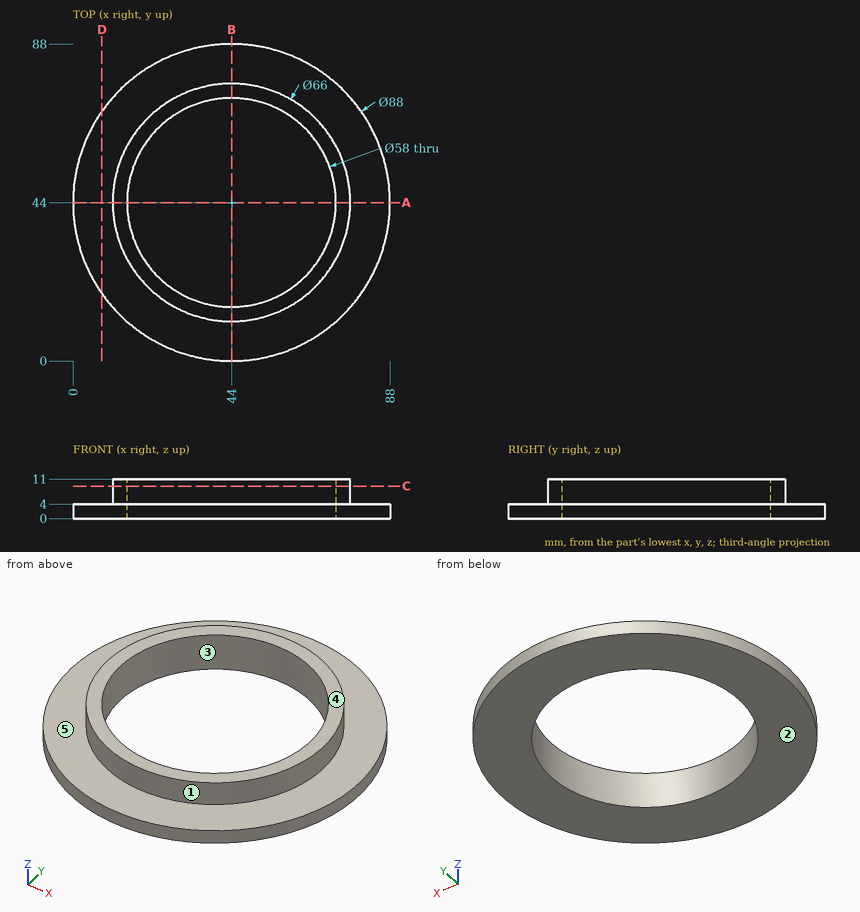
For this review, use the dimensioned drawing (mm, ordinates from the lowest corner) and the shaded views. A direction names the side the tool comes from. Coordinates: 2 decimals unless noted, no trailing zeros. Loops run counter-clockwise (first coordinate to the right, second up) from the corner with the lowest first, then second, coordinate; pieces in that order, holes last.
1. Add section D-D, the plane x = 8. Give the boundary of the cut face in (y, z), then the cut area to 3 significant figures.
2. Insertion check: P1, Ø4, axis at x = 72.5, y = 16, coming from the +Z side; P2, Ø1.5, axis at x = 16, y = 66.5, coming from the -Z side; P3, Ø4, axis at y = 23, z = 1.5, coming from the -X side; P4, Ø6, axis at y = 60.5, z = 7.5, coming from the -X side. Each pin has a flat end and moves straight along its axis. Give the tip position at first contact, or say it passes through.
3. Add section C-C, the plane z = 9. Give the boundary of the cut face in (x, y), then the cut area to 3 significant figures.
4. Mouldability with a two-part tool opening along X and no side actions: class the marked faces 1, 2 and 3 as +X half, -X half, draft (parallel to the pull), parting line (faces both ways), or undercut.
5. Add section A-A, the plane y = 44. Give the boundary of the cut face in (x, z), then the cut area to 3 significant figures.
6. For line 1 (Z direction, x = 7.5, y = 59.5); line 2 (Y direction, x = 32, z = 2.5); line 3 (Y direction, x = 44, z = 2), list the stretches that pass through material, from the lowest coordinate up.
7. For the marked faces 4 and 5, list the 3-axis set-ups (+Z, -Z, +X, -X, +Y, -Y) from which the entire face can be reached by the end or side of a thin tool; tool diameter is ignored.
Result:
1. outline: (18.7, 0) - (69.3, 0) - (69.3, 4) - (18.7, 4) - close
1. area: 202 mm2
2. P1: stops at z = 4
2. P2: stops at z = 0
2. P3: stops at x = 4.31
2. P4: stops at x = 13.89
3. outline: circle Ø66 at (44, 44); hole circle Ø58 at (44, 44)
3. area: 779 mm2
4. face 1: parting line
4. face 2: draft
4. face 3: undercut
5. outline: (0, 0) - (15, 0) - (15, 11) - (11, 11) - (11, 4) - (0, 4) - close; (73, 0) - (88, 0) - (88, 4) - (77, 4) - (77, 11) - (73, 11) - close
5. area: 176 mm2
6. line 1: z = 0 to 4
6. line 2: y = 1.67 to 17.6, 70.4 to 86.33
6. line 3: y = 0 to 15, 73 to 88
7. face 4: +Z, +X, -X, +Y, -Y
7. face 5: +Z
